```python
from build123d import *
from build123d.topology import SkipClean

# Parameters (mm, degrees)
SZKIC2_R                        = 2.5
DODANIE_WYCI_GNI_CIE1_DEPTH     = 30
WYTNIJ_WYCI_GNI_CIE1_DEPTH      = 20
WYTNIJ_WYCI_GNI_CIE1_DEPTH_BACK = 20


with BuildPart() as part:
    # Szkic2 → Dodanie-wyci_gni_cie1 (new body)
    with BuildSketch(Plane(origin=(0, 0, 0), x_dir=(1, 0, 0), z_dir=(0, 1, 0))):
        with Locations(Location((0, 0, 0), (0, 0, 270))):
            Circle(SZKIC2_R)
    extrude(amount=DODANIE_WYCI_GNI_CIE1_DEPTH)

    # Szkic3 → Obr_t2 (revolve)
    with BuildSketch(Plane.XY, mode=Mode.PRIVATE) as obr_t2_sk:
        with BuildLine():
            ThreePointArc((-1.081563109, 32), (-0.764780609, 31.235219391), (0, 30.918436891))
            Line((0, 30.918436891), (0, 32))
            Line((0, 32), (0, 39))
            Line((0, 39), (0, 40))
            Line((0, 40), (0, 40.081563109))
            ThreePointArc((0, 40.081563109), (-0.764780609, 39.764780609), (-1.081563109, 39))
            Line((-1.081563109, 39), (-1.081563109, 32))
        make_face()
        with BuildLine():
            Line((-2.497718644, 41), (-2.497718644, 30))
            Line((-2.497718644, 30), (0, 30))
            Line((0, 30), (0, 30.918436891))
            ThreePointArc((0, 30.918436891), (-0.764780609, 31.235219391), (-1.081563109, 32))
            Line((-1.081563109, 32), (-1.081563109, 39))
            ThreePointArc((-1.081563109, 39), (-0.764780609, 39.764780609), (0, 40.081563109))
            Line((0, 40.081563109), (0, 41))
            Line((0, 41), (0, 43.497718644))
            ThreePointArc((0, 43.497718644), (-1.766153791, 42.766153791), (-2.497718644, 41))
        make_face()
    revolve(obr_t2_sk.sketch.rotate(Axis((0, 0, 0), (0, 1, 0)), 180), axis=Axis((0, 0, 0), (0, 1, 0)))

    # Szkic3_3 → Wytnij-wyci_gni_cie1 (cut, two sides: drawn at the far end of the back side and taken through both)
    with BuildSketch(Plane.XY.offset(-WYTNIJ_WYCI_GNI_CIE1_DEPTH_BACK)):
        with BuildLine():
            ThreePointArc((-1.081563109, 32), (-0.764780609, 31.235219391), (0, 30.918436891))
            Line((0, 30.918436891), (0, 32))
            Line((0, 32), (0, 39))
            Line((0, 39), (0, 40))
            Line((0, 40), (0, 40.081563109))
            ThreePointArc((0, 40.081563109), (-0.764780609, 39.764780609), (-1.081563109, 39))
            Line((-1.081563109, 39), (-1.081563109, 32))
        make_face()
        with BuildLine():
            Line((0, 32), (0, 30.918436891))
            ThreePointArc((0, 30.918436891), (0.764780609, 31.235219391), (1.081563109, 32))
            Line((1.081563109, 32), (1.081563109, 39))
            ThreePointArc((1.081563109, 39), (0.764780609, 39.764780609), (0, 40.081563109))
            Line((0, 40.081563109), (0, 40))
            Line((0, 40), (0, 39))
            Line((0, 39), (0, 32))
        make_face()
    extrude(amount=WYTNIJ_WYCI_GNI_CIE1_DEPTH + WYTNIJ_WYCI_GNI_CIE1_DEPTH_BACK, mode=Mode.SUBTRACT)

    # Szkic4 → Obr_t3 (revolve)
    with SkipClean():  # the faces are left unmerged after this step: merging them gives an invalid solid
        with BuildSketch(Plane.XY):
            with BuildLine():
                ThreePointArc((-2.5, 0), (-1.382027756, -0.869452827), (0, -1.178983829))
                Line((0, -1.178983829), (0, 0))
                Line((0, 0), (-2.5, 0))
            make_face()
            with BuildLine():
                Line((0, 0), (0, -1.178983829))
                ThreePointArc((0, -1.178983829), (1.382027756, -0.869452827), (2.5, 0))
                Line((2.5, 0), (0, 0))
            make_face()
        revolve(axis=Axis((0, -1.178983829, 0), (0, 1, 0)))
    add(part.part.scale(1), mode=Mode.REPLACE)  # the faces are merged on a copy


solid = part.part
```
Build history of the part. All positions in model axes, mm. A direction names the side the tool comes from. Give positions to 0.01 mm unless a question says otherwise; leave off trailing zeros. Loops run counter-clockwise (first coordinate to the right, second up) from the corner with the lowest first, then second, coordinate; pieces in that order, holes last. Notation, with made-up numbers: (9.5, 82) - (64.5, 82) arc R15 cw to (64.5, 87) - close; hole circle Ø2 at (27, 11.25). An arc over 180 degrees is marked (long way). Use a Markdown table: item, result.
(1) Band-saw the part on C-C (y = 29.5). Give the cut face in (x, z).
Taken from the geometry:
| item | result |
|---|---|
| outline | circle Ø5 at (0, 0) |
(2) Drop flat-ended pins along their axis: pin 1 Ø1.4 at (y, z) = (36, 0.5) entering from +X; pin 2 Ø2 at (y, z) = (14, 1.5) entering from +X; pin 3 Ø1.5 at (x, z) = (0.5, 1) entering from +Y. Give the stop position or say it passes through.
Taken from the geometry:
| item | result |
|---|---|
| pin 1 | x = 2.5 |
| pin 2 | x = 2.45 |
| pin 3 | y = 43.47 |
(3) Band-saw the part on B-B (y = 34). Give the cut face in (x, z), and give its area (3 significant figures).
Taken from the geometry:
| item | result |
|---|---|
| outline | (-1.08, -2.25) - (-1.08, 2.25) arc R2.5 ccw to start; (1.08, -2.25) arc R2.5 ccw to (1.08, 2.25) - close |
| area | 9.14 mm2 |
(4) Wall check: line 1 along X through (y, z) = (28.5, 1.1) (3 decimals); line 2 along Z through (x, y) = (0.1, 21.5); line 3 along X through (y, z) = (18, 2.1). Give the ranges that are in metal, low to high.
Taken from the geometry:
| item | result |
|---|---|
| line 1 | -2.245 to 2.245 |
| line 2 | -2.5 to 2.5 |
| line 3 | -1.36 to 1.36 |
(5) Pull direction Y, two halves, no side cores. Call faces 1 (the face through (-2.44, 14.79, -0.54)), 2 (the face through (-1.082, 36, 0)): +Y half, -Y half, draft (parallel to the pull), parting line (faces both ways), or undercut.
Taken from the geometry:
| item | result |
|---|---|
| face 1 | draft |
| face 2 | undercut |
(6) Which spindle directions (+Z, -Z, +X, -X, +Y, -Y) get a long thin tool onto all of the face, cutting with end or side? Do faces 3 (the face through (2.382, 35.423, -0.75)), 4 (the face through (1.082, 35, 0)). Say none if no direction does.
Taken from the geometry:
| item | result |
|---|---|
| face 3 | +Y, -Y |
| face 4 | +Z, -Z |
